Autodesk Inventor part; units mm, degrees
ref_plane "YZ Plane" through (0, 0, 0) normal (1, 0, 0) x (0, 1, 0)
ref_plane "XZ Plane" through (0, 0, 0) normal (0, 1, 0) x (-1, 0, 0)
ref_plane "XY Plane" through (0, 0, 0) normal (0, 0, 1) x (1, 0, 0)
sketch "Sketch1" plane through (0, 0, 0) normal (0, 1, 0) x (-1, 0, 0)
  line L0 (0, 0) -> (24, 0)
  line L1 (24, 0) -> (24, -24)
  line L2 (24, -24) -> (0, -24)
  line L3 (0, -24) -> (0, 0)
  dimension "d0" = 24
  dimension "d1" = 24
extrude "Extrusion1" add sketch "Sketch1" along normal blind 2
sketch "Sketch2" plane through (0, 2, 0) normal (0, 1, 0) x (1, 0, 0)
  line L0 (0, 24) -> (-24, 24)
  line L1 (-24, 0) -> (0, 0)
  line L2 (-24, 24) -> (0, 0)
  line L3 (0, 24) -> (-24, 0)
  line L4 (-17, 17) -> (-7, 17)
  line L5 (-7, 17) -> (-7, 7)
  line L6 (-7, 7) -> (-17, 7)
  line L7 (-17, 7) -> (-17, 17)
  line L8 (-17, 17) -> (-7, 7) construction
  line L9 (-7, 17) -> (-17, 7) construction
  point P0 (-12, 12)
  point P1 (-12, 12)
  dimension "d4" = 10
extrude "Extrusion2" cut sketch "Sketch2" against normal through all contours L5 L2 L3 | L3 L2 L4 | L2 L3 L7 | L2 L6 L3
fillet "Fillet1" radius 2 8 edges at (0, 1, 0) (0, 1, -24) (-24, 1, 0) (-24, 1, -24) (-7, 1, -17) (-17, 1, -17) (-17, 1, -7) (-7, 1, -7)
properties part number "hot_glue_mashroom"
Source: CAD feature listing. Evaluate the final solid. Frame: model axes, mm. A direction names the side the tool comes from. Give positions to 0.01 mm unless a question says otherwise; leave off trailing zeros. Order: outer loops, then holes, each group sorted by start corner. A loop starts at its lowest first (then second) coordinate and runs counter-clockwise, first axis right, second up.
(1) Access query for faces 1 (the face through (-24, 1, -12)), 2 (the face through (-16.43, 0.99, -16.4)). Directions: +Z, -Z, +X, -X, +Y, -Y. A direction counts if a zero-diameter tool reaches every point of the face in a straight line with its end or side. Return the directions, or none.
(2) Section query B-B (z = -10.75). Return the cut outline in (x, y), plus the area to 3 significant figures.
(3) Material intervals for line 1 along X through (y, z) = (1.75, -9); line 2 along Z through (x, y) = (-16, 0.2), sorted ascending.
(4) Section query A-A (x = -10). Return the cut outline in (y, z), plus the area to 3 significant figures.
(5) Pull-direction query (X, two-part tool) for faces 3 (the face through (-23.4, 1.01, -23.43)), 4 (the face through (-12, 1, -7)), 5 (the face through (-12, 1, -24)); classes: +X half, -X half, draft (parallel to the pull), parting line (faces both ways), or undercut.
(6) Section query C-C (y = 0.95). Return the cut outline in (x, z).
Outcome:
1. face 1: +Z, -Z, -X, +Y, -Y
1. face 2: +Y, -Y
2. outline: (-24, 0) - (-17, 0) - (-17, 2) - (-24, 2) - close; (-7, 0) - (0, 0) - (0, 2) - (-7, 2) - close
2. area: 28.0 mm2
3. line 1: x = -24 to -17, -7 to 0
3. line 2: z = -24 to -16.73, -7.27 to 0
4. outline: (0, -24) - (2, -24) - (2, -17) - (0, -17) - close; (0, -7) - (2, -7) - (2, 0) - (0, 0) - close
4. area: 28.0 mm2
5. face 3: -X half
5. face 4: undercut
5. face 5: draft
6. outline: (-24, -22) arc R2 ccw to (-22, -24) - (-2, -24) arc R2 ccw to (0, -22) - (0, -2) arc R2 ccw to (-2, 0) - (-22, 0) arc R2 ccw to (-24, -2) - close; hole (-17, -15) arc R2 ccw to (-15, -17) - (-9, -17) arc R2 ccw to (-7, -15) - (-7, -9) arc R2 ccw to (-9, -7) - (-15, -7) arc R2 ccw to (-17, -9) - close
